```python
from build123d import *

# Parameters (mm, degrees)
F0_W     = 1219.2
F0_H     = 1219.2
F1_DEPTH = 1219.2
F2_T     = -2.54
F4_DEPTH = 1219.2


with BuildPart() as f1:
    # F0 (on Top) → F1 (new body)
    with BuildSketch(Plane.XY):
        Rectangle(F0_W, F0_H)
    extrude(amount=F1_DEPTH)

    # F2
    f2_openings = [f1.faces().sort_by_distance(p)[0] for p in [
        (0, 0, 1219.2),
    ]]
    offset(amount=F2_T, openings=f2_openings)

    # F3 (on face) → F4 (cut)
    with BuildSketch(Plane(origin=(-609.6, 0, 0), x_dir=(0, -1, 0), z_dir=(-1, 0, 0))):
        Polygon((609.6, 836.845815), (609.6, 1219.2), (304.8, 1219.2), align=None)
    extrude(amount=-F4_DEPTH, mode=Mode.SUBTRACT)


solid = f1.part
```
Part model, mm, in its own coordinate system. A direction names the side the tool comes from. Coordinates: 2 decimals unless noted, no trailing zeros. Loops run counter-clockwise (first coordinate to the right, second up) from the corner with the lowest first, then second, coordinate; pieces in that order, holes last. Notation, with made-up numbers: (-40, 77.5) - (-32, 77.5) arc R21 ccw to (-32, 115.5) - close; hole circle Ø7 at (4, 68.25). An arc over 180 degrees is marked (long way). Write item = value, one per line. Start each with the question number.
Item 1: 3-axis set-ups, long thin cutter, end or side, ignore diameter. For faces 1 (the flat face through (609.6, -9, 601)), 2 (the flat face through (-8, 607.06, 602)): which of +Z, -Z, +X, -X, +Y, -Y reach the whole face in a straight line?
Item 2: Cut at A-A, the plane z = 657.5. Give the cut face in (x, y), and give its area (3 significant figures).
Item 3: Wall check: L1, parallel to X at y = 128.5, z = 593.5; L2, parallel to Z at x = -332, y = 437.5. Give the ranges that are in metal, low to high. Write a range as from..to.
Item 4: Cut at B-B, the plane y = -216. Give the cut face in (x, z).
Item 5: Cut at C-C, the plane x = 448.5. Give the cut face in (y, z), and give its area (3 significant figures).
Item 6: Flat gauge pin, fed straight in: pin 1 Ø8 at (x, y) = (-418.5, -5.5) entering from +Z. Where does the tip first touch, or does it go through?
Item 7: Mould opens along X. For faces 3 (the flat face through (-8, 8, 2.54)), 4 (the flat face through (-609.6, -9, 601)), 5 (the flat face through (-9, 609.6, 601)) say: released by +X, released by -X, zero draft, split by the parting line, or undercut.
The answers:
q1.face_1 = +Z, -Z, +X, +Y, -Y
q1.face_2 = +Z
q2.outline = (-609.6, -609.6) - (609.6, -609.6) - (609.6, 609.6) - (-609.6, 609.6) - close; hole (-607.06, -607.06) - (607.06, -607.06) - (607.06, 607.06) - (-607.06, 607.06) - close
q2.area = 12,400 mm2
q3.L1 = -609.6..-607.06, 607.06..609.6
q3.L2 = 0..2.54
q4.outline = (-609.6, 0) - (609.6, 0) - (609.6, 1219.2) - (607.06, 1219.2) - (607.06, 2.54) - (-607.06, 2.54) - (-607.06, 1219.2) - (-609.6, 1219.2) - close
q5.outline = (-609.6, 0) - (609.6, 0) - (609.6, 1219.2) - (607.06, 1219.2) - (607.06, 2.54) - (-607.06, 2.54) - (-607.06, 840.03) - (-609.6, 836.85) - close
q5.area = 8,310 mm2
q6.pin_1 = 2.54
q7.face_3 = undercut
q7.face_4 = released by -X
q7.face_5 = zero draft
